The listing builds one solid part. Answer for the finished solid, in the listing's coordinates (mm). Coordinates: 2 decimals unless noted, no trailing zeros. Order: outer loops, then holes, each group sorted by start corner. A loop starts at its lowest first (then second) coordinate and runs counter-clockwise, first axis right, second up. Notation, with made-up numbers: (60, -34) -> (109, -34) arc R11 ccw to (109, -25) -> close; hole circle Ø4 at (-18, -34). An arc over 180 degrees is marked (long way). Return JSON: item names as keys, results as strings.
Autodesk Inventor part; units mm, degrees
ref_plane "YZ Plane" through (0, 0, 0) normal (1, 0, 0) x (0, 1, 0)
ref_plane "XZ Plane" through (0, 0, 0) normal (0, 1, 0) x (-1, 0, 0)
ref_plane "XY Plane" through (0, 0, 0) normal (0, 0, 1) x (1, 0, 0)
sketch "Sketch1" plane through (0, 0, 0) normal (0, 0, 1) x (1, 0, 0)
  circle A0 centre (0, 0) radius 1
  circle A1 centre (-23.2, 0) radius 1
  line L0 (-23.2, 2) -> (0, 2)
  arc A2 (0, -2) -> (0, 2) centre (0, 0) ccw
  line L1 (0, -2) -> (-23.2, -2)
  arc A3 (-23.2, 2) -> (-23.2, -2) centre (-23.2, 0) ccw
  dimension "d0" = 2
  dimension "d1" = 23.2
  dimension "d2" = 2
extrude "Extrusion1" add sketch "Sketch1" along normal blind 2
properties part number "panto_linkageB"
Item 1: The part is cut by section A-A on z = 1. Determine the outline of the cut face in (x, y), plus the area to 3 significant figures.
Answer list:
{"outline": "(-23.2, -2) -> (0, -2) arc R2 ccw to (0, 2) -> (-23.2, 2) arc R2 ccw to start; hole circle Ø2 at (-23.2, 0); hole circle Ø2 at (0, 0)", "area": "99.1 mm2"}
Item 2: The part is cut by section B-B on y = 0. Determine the outline of the cut face in (x, z).
Answer list:
{"outline": "(-25.2, 0) -> (-24.2, 0) -> (-24.2, 2) -> (-25.2, 2) -> close; (-22.2, 0) -> (-1, 0) -> (-1, 2) -> (-22.2, 2) -> close; (1, 0) -> (2, 0) -> (2, 2) -> (1, 2) -> close"}
Item 3: Determine the mould class of faces 1 (the flat face through (-12, 0, 2)), 2 (the cylindrical face through (0, 1, 1)), 3 (the flat face through (-12, 2, 1)) for opening direction Y: pulls with the +Y half, pulls with the -Y half, needs draft (parallel to the pull), parting line crosses it, or undercut.
Answer list:
{"face 1": "needs draft", "face 2": "undercut", "face 3": "pulls with the +Y half"}
Item 4: Find the intervals of material crossed by probe 1 along Y at (x, z) = (0, 1.5); probe 2 along X at (y, z) = (0.65, 0.5); probe 3 along X at (y, z) = (-1.5, 0.5), in increasing order.
Answer list:
{"probe 1": "-2 to -1, 1 to 2", "probe 2": "-25.09 to -23.96, -22.44 to -0.76, 0.76 to 1.89", "probe 3": "-24.52 to 1.32"}
